Job drawing, mm, ordinate dimensions from the low corner. One solid piece. Give positions to 0.01 mm unless a question says otherwise; leave off trailing zeros. Order: outer loops, then holes, each group sorted by start corner. A loop starts at its lowest first (then second) coordinate and runs counter-clockwise, first axis right, second up. Notation, with made-up numbers: (8, -21) - (44, -21) arc R22 cw to (44, -8) - close; hole circle Ø5 at (-27.75, 5.5). An arc over 180 degrees is marked (long way). One line per item, written item: value.
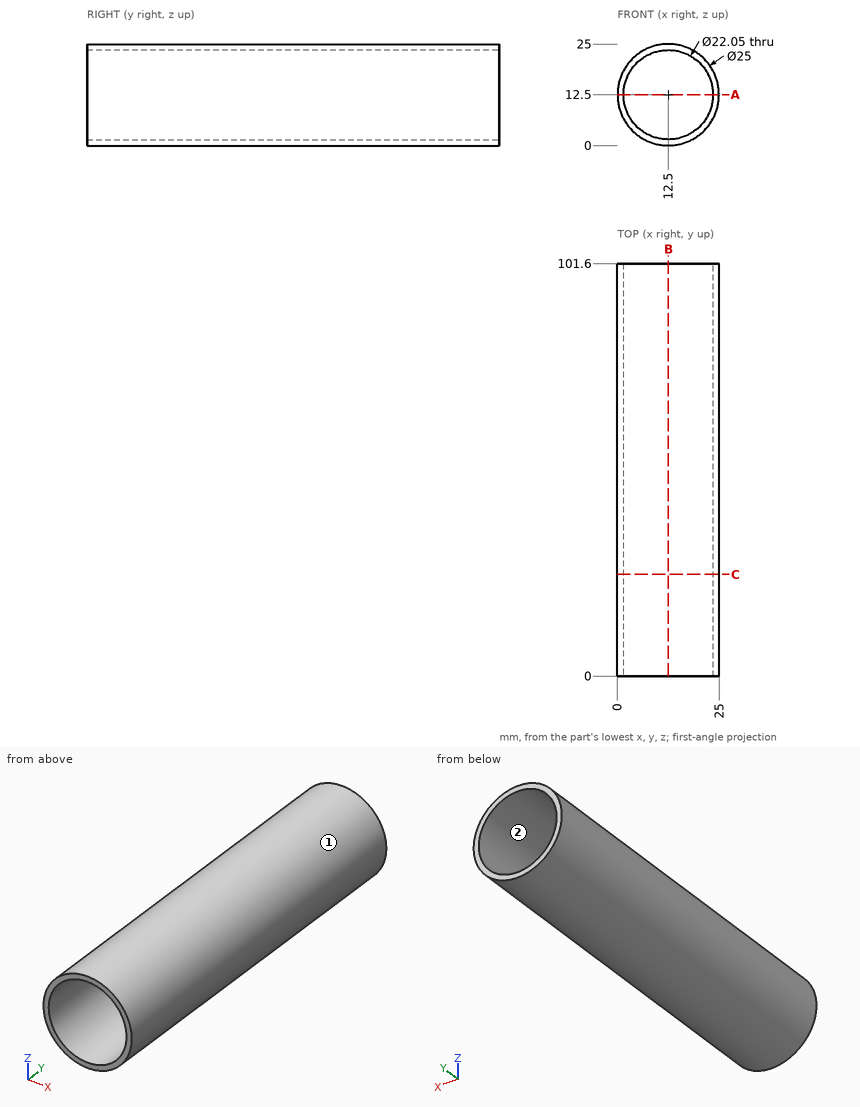
1) Wall check: line 1 along Z through (x, y) = (12.5, 40) (3 decimals); line 2 along X through (y, z) = (19.5, 19.75); line 3 along Z through (x, y) = (10.25, 83). Give the ranges that are in metal, low to high. Write a range as [from, to].
Answer:
line 1: z = [0, 1.475], [23.525, 25]
line 2: x = [2.32, 4.19], [20.81, 22.68]
line 3: z = [0.2, 1.71], [23.29, 24.8]
2) Two-plate mould, pull along X, no slides. Class the marked faces 1 and 2: pulls with the +X half, pulls with the -X half, needs draft (parallel to the pull), parting line crosses it, or undercut.
Answer:
face 1: parting line crosses it
face 2: undercut
3) Drop flat-ended pins along their axis: P1, Ø4, axis at x = 6.5, y = 64.5, coming from the +Z side; P2, Ø12, axis at y = 39, z = 14, coming from the +X side; P3, Ø4, axis at y = 85.5, z = 6, coming from the -X side; P4, Ø12, axis at x = 10, z = 9.5, coming from the -Y side. Give the stop position or say it passes through.
Answer:
P1: stops at z = 24.34
P2: stops at x = 25
P3: stops at x = 0.84
P4: passes through
4) Slice it at C-C on y = 25. Write the cut outline in (x, z) (3 decimals), then the cut area to 3 significant figures.
Answer:
outline: circle Ø25 at (12.5, 12.5); hole circle Ø22.05 at (12.5, 12.5)
area: 109 mm2
5) Slice it at A-A on z = 12.5. Write the cut outline in (x, y) (3 decimals).
Answer:
outline: (0, 0) - (1.475, 0) - (1.475, 101.6) - (0, 101.6) - close; (23.525, 0) - (25, 0) - (25, 101.6) - (23.525, 101.6) - close
6) Slice it at B-B on x = 12.5. Write the cut outline in (y, z) (3 decimals).
Answer:
outline: (0, 0) - (101.6, 0) - (101.6, 1.475) - (0, 1.475) - close; (0, 23.525) - (101.6, 23.525) - (101.6, 25) - (0, 25) - close
